Part print with two shaded views. Sizes in mm from the minimum x, y, z corner. Round coordinates to 2 decimals unless told otherwise and drop trailing zeros. Answer as a JSON object with one key per item and string values. Group by question number.
Item 1: Flat gauge pin, fed straight in: pin 1 (4 mm diameter, centred on x = 15.875, z = 12.7, fed in from -Y). Where does the tip first touch, or does it go through?
Item 2: Probe line 1 (Z direction, x = 169, y = 4.1); line 2 (Z direction, x = 91.5, y = 3.8). List the from-to ranges inside material, lowest first. Write a range as from..to.
Item 3: Slice it at A-A, the plane y = 3.9. Give the number of separate pieces and of enclosed holes in the cut face, then the cut area to 3 significant figures.
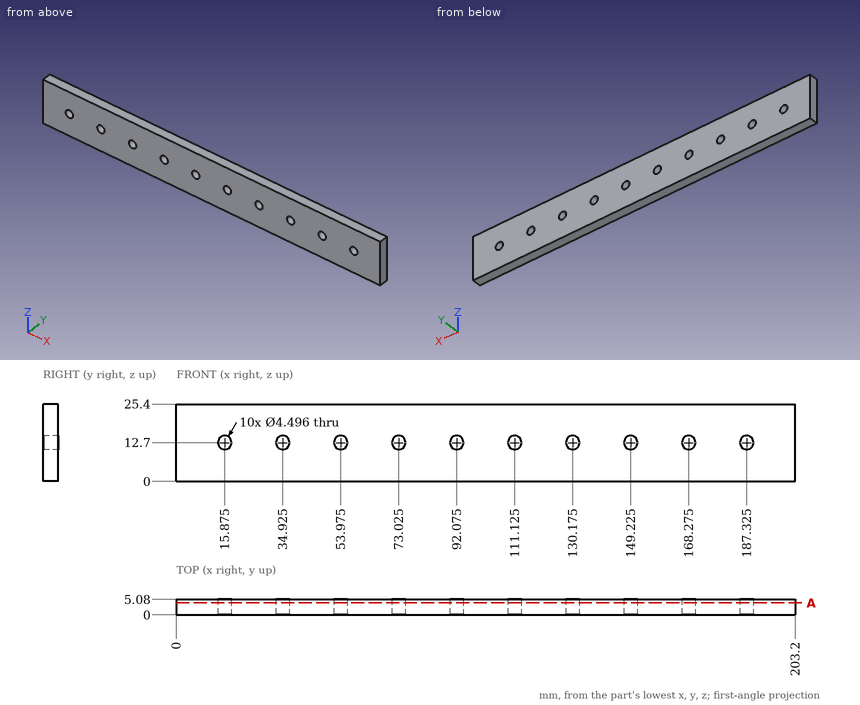
Geometry says:
{
 "1": {"pin 1": "passes through"},
 "2": {"line 1": "z = 0..10.57, 14.83..25.4", "line 2": "z = 0..10.53, 14.87..25.4"},
 "3": {"separate pieces": "1", "enclosed holes": "10", "area": "5,000 mm^2"}
}
